from build123d import *

# Parameters (mm, degrees)
F0_W        = 39.9140380323
F0_H        = 79.8528119922
F1_DEPTH    = 12.7
F2_T1_DEPTH = 170.555533821
F3_R        = 5.08
F4_SIZE     = 5.08
F5_R        = 11.650994652


# Not quite as in the source:
# - a fillet or chamfer that OpenCascade refuses, or shapes differently, is made with other operations: its cross-section is extruded or revolved along the edge and cut away or added


with BuildPart() as f1:
    # F0 (on Top) → F1 (new body)
    with BuildSketch(Plane.XY):
        with Locations((0, -6.916385144)):
            Rectangle(F0_W, F0_H)
    extrude(amount=F1_DEPTH)

    # F2: chamfer of 25.4 on 1 edges, made by hand

    # F2_s2 → F2_t1 (cut)
    with BuildSketch(Plane.YZ.offset(-85.2777669105)):
        Polygon((33.0100208521, -12.7), (7.6100208521, 12.7), (33.0100208521, 12.7), align=None)
    extrude(amount=F2_T1_DEPTH, mode=Mode.SUBTRACT)

    # F3
    f3_edges = [f1.edges().sort_by_distance(p)[0] for p in [
        (19.957019, -13.266385, 0),
        (-19.957019, -13.266385, 0),
    ]]
    fillet(f3_edges, radius=F3_R)

    # F4
    f4_edges = [f1.edges().sort_by_distance(p)[0] for p in [
        (-19.957019, -19.616385, 12.7),
        (19.957019, -19.616385, 12.7),
    ]]
    chamfer(f4_edges, length=F4_SIZE)

    # F5
    f5_edges = [f1.edges().sort_by_distance(p)[0] for p in [
        (0, -46.842791, 12.7),
    ]]
    fillet(f5_edges, radius=F5_R)


solid = f1.part
Part model, mm, in its own coordinate system. Coordinates: 2 decimals unless noted, no trailing zeros. Order: outer loops, then holes, each group sorted by start corner. A loop starts at its lowest first (then second) coordinate and runs counter-clockwise, first axis right, second up.
(1) Slice it at B-B, the plane x = 7.5. Write the cut outline in (y, z), and give its area (3 significant figures).
Check sheet entries:
outline: (-46.84, 0) - (20.31, 0) - (7.61, 12.7) - (-35.19, 12.7) arc R11.65 ccw to (-46.84, 1.05) - close
area: 743 mm2
(2) Probe L1, parallel to X at y = -38.5, z = 9.5; L2, parallel to X at y = -41.5, z = 2.5; L3, parallel to Z at x = -17, y = -39. List the from-to ranges inside material, lowest first.
Check sheet entries:
L1: x = -18.08 to 18.08
L2: x = -19.25 to 19.25
L3: z = 0.46 to 10.58
(3) Slice it at C-C, the plane z = 9.25. Write the cut outline in (x, y).
Check sheet entries:
outline: (-18.33, -43.47) - (18.33, -43.47) - (18.33, 11.06) - (-18.33, 11.06) - close
(4) Slice it at D-D, the plane y = 11. Write the cut outline in (x, z).
Check sheet entries:
outline: (-19.96, 5.08) arc R5.08 ccw to (-14.88, 0) - (14.88, 0) arc R5.08 ccw to (19.96, 5.08) - (19.96, 7.62) - (18.27, 9.31) - (-18.27, 9.31) - (-19.96, 7.62) - close
(5) Slice it at A-A, the plane y = -12. Write the cut outline in (x, z), and give its area (3 significant figures).
Check sheet entries:
outline: (-19.96, 5.08) arc R5.08 ccw to (-14.88, 0) - (14.88, 0) arc R5.08 ccw to (19.96, 5.08) - (19.96, 7.62) - (14.88, 12.7) - (-14.88, 12.7) - (-19.96, 7.62) - close
area: 470 mm2
(6) Pin check, flat tips, straight feed: pin 1 Ø5 at (x, z) = (6.5, 10) entering from -Y; pin 2 Ø1 at (x, z) = (-7.5, 7.5) entering from -Y; pin 3 Ø2 at (x, y) = (2.5, 10) entering from +Z. Stop position of each tip, or through.
Check sheet entries:
pin 1: stops at y = -44.89
pin 2: stops at y = -45.21
pin 3: stops at z = 11.31
